from build123d import *

# Parameters (mm, degrees)
BOSS_EXTRUDE1_DEPTH = 12.5
SKETCH4_OUTSIDE_W   = 62.868
SKETCH4_OUTSIDE_H   = 25.468
SKETCH4_OUTSIDE_R   = 5
CUT_EXTRUDE6_DEPTH  = 9.11
SKETCH5_R           = 3
CUT_EXTRUDE7_DEPTH  = 9.11
CUT_EXTRUDE8_REACH  = 21.017
SKETCH6_R           = 2.5


with BuildPart() as part:
    # Sketch1 → Boss-Extrude1 (new body)
    with BuildSketch(Plane.XY):
        with BuildLine():
            Line((-10.816653826, 19.01731952), (-19.949874371, 19.01731952))
            Line((-19.949874371, 19.01731952), (-24.949874371, 19.01731952))
            Line((-24.949874371, 19.01731952), (-24.949874371, 17.01731952))
            Line((-24.949874371, 17.01731952), (-19.949874371, 17.01731952))
            Line((-19.949874371, 17.01731952), (-12.369316877, 17.01731952))
            ThreePointArc((-12.369316877, 17.01731952), (-11.780968471, 16.82592706), (-11.417830963, 16.325011828))
            ThreePointArc((-11.417830963, 16.325011828), (-8.966906745, 12.042698311), (-5, 9.108607405))
            Line((-5, 9.108607405), (-5, 0))
            Line((-5, 0), (5, 0))
            Line((5, 0), (5, 9.108607405))
            ThreePointArc((5, 9.108607405), (8.966906745, 12.042698311), (11.417830963, 16.325011828))
            ThreePointArc((11.417830963, 16.325011828), (11.780968471, 16.82592706), (12.369316877, 17.01731952))
            Line((12.369316877, 17.01731952), (19.949874371, 17.01731952))
            Line((19.949874371, 17.01731952), (24.949874371, 17.01731952))
            Line((24.949874371, 17.01731952), (24.949874371, 19.01731952))
            Line((24.949874371, 19.01731952), (19.949874371, 19.01731952))
            Line((19.949874371, 19.01731952), (10.816653826, 19.01731952))
            ThreePointArc((10.816653826, 19.01731952), (10.177051677, 18.786025635), (9.83332166, 18.199137702))
            ThreePointArc((9.83332166, 18.199137702), (0, 10.01731952), (-9.83332166, 18.199137702))
            ThreePointArc((-9.83332166, 18.199137702), (-10.177051677, 18.786025635), (-10.816653826, 19.01731952))
        make_face()
    extrude(amount=BOSS_EXTRUDE1_DEPTH)

    # Sketch4 outside → Cut-Extrude6 (cut)
    with BuildSketch(Plane.XZ):
        with Locations((0, 6.25)):
            Rectangle(SKETCH4_OUTSIDE_W, SKETCH4_OUTSIDE_H)
        with Locations((0, 6.25)):
            Circle(SKETCH4_OUTSIDE_R, mode=Mode.SUBTRACT)
    extrude(amount=-CUT_EXTRUDE6_DEPTH, mode=Mode.SUBTRACT)

    # Sketch5 → Cut-Extrude7 (cut)
    with BuildSketch(Plane.XZ):
        with Locations((0, 6.25)):
            Circle(SKETCH5_R)
    extrude(amount=-CUT_EXTRUDE7_DEPTH, mode=Mode.SUBTRACT)

    # Sketch6 → Cut-Extrude8 (cut, up to next)
    with BuildSketch(Plane(origin=(0, 19.01731952, 0), x_dir=(1, 0, 0), z_dir=(0, 1, 0)), mode=Mode.PRIVATE) as cut_extrude8_sk1:
        with Locations((-18.699874371, -6.25)):
            Circle(SKETCH6_R)
    cut_extrude8_tool1 = extrude(cut_extrude8_sk1.sketch, amount=-CUT_EXTRUDE8_REACH, mode=Mode.PRIVATE) & part.part
    add(cut_extrude8_tool1.solids().sort_by_distance((-18.699874, 19.01732, 6.25))[0], mode=Mode.SUBTRACT)
    # Sketch6 → Cut-Extrude8 (cut, up to next)
    with BuildSketch(Plane(origin=(0, 19.01731952, 0), x_dir=(1, 0, 0), z_dir=(0, 1, 0)), mode=Mode.PRIVATE) as cut_extrude8_sk2:
        with Locations((18.699874371, -6.25)):
            Circle(SKETCH6_R)
    cut_extrude8_tool2 = extrude(cut_extrude8_sk2.sketch, amount=-CUT_EXTRUDE8_REACH, mode=Mode.PRIVATE) & part.part
    add(cut_extrude8_tool2.solids().sort_by_distance((18.699874, 19.01732, 6.25))[0], mode=Mode.SUBTRACT)


solid = part.part
The model under review builds one solid part; all positions refer to its coordinate system, in mm. A direction names the side the tool comes from. Give positions to 0.01 mm unless a question says otherwise; leave off trailing zeros. Write each loop counter-clockwise with the first axis right and the second up, starting at its lowest first coordinate (ties: lowest second). Pieces come first, ordered by that corner, then holes.
1. Add section A-A, the plane z = 6.25. Count the separate pieces of the cut face and the enclosed holes in it, plus the area to 3 significant figures.
2. For P1, Ø4, axis at x = -19, z = 8, coming from the -Y side; P2, Ø5, axis at x = 0, z = 6.25, coming from the -Y side, all flat-tipped, find the tip position at first contact; note any pin that passes through.
3. Add section D-D, the plane y = 8.25. Write out the cut boundary in (x, z).
4. Draft analysis for pull direction X (two halves, no side actions). For faces 4 (the flat face through (19, 17.017, 3)), 5 (the cylindrical face through (21.01, 18.03, 7.21)), 6 (the cylindrical face through (-0.65, 4.49, 3.32)), 7 (the flat face through (-24.95, 18, 6)), state which applies: +X half, -X half, draft (parallel to the pull), parting line (faces both ways), or undercut.
5. Add section B-B, the plane x = 0. Write out the cut boundary in (y, z).
6. Add section C-C, the plane x = 18. Write out the cut boundary in (y, z).
7. Tool access review of faces 1 (the flat face through (-19, 17.017, 3)), 2 (the cylindrical face through (-1.08, 4.49, 1.37)), 3 (the cylindrical face through (-10.17, 18.78, 6.16)): name each direction out of +Z, -Z, +X, -X, +Y, -Y from which nothing blocks a thin tool from reaching the whole face with its end or side.
8. Wall thickness on L1, parallel to Z at x = 0, y = 4.75; L2, parallel to Y at x = 20, z = 2.75; L3, parallel to X at y = 17.45, z = 6.25: over which ranges is each line inside the solid? List them lowest first.
Worked answers:
1. separate pieces: 3
1. enclosed holes: 0
1. area: 127 mm2
2. P1: stops at y = 17.02
2. P2: stops at y = 9.11
3. outline: circle Ø10 at (0, 6.25); hole circle Ø6 at (0, 6.25)
4. face 4: draft
4. face 5: undercut
4. face 6: undercut
4. face 7: -X half
5. outline: (0, 1.25) - (9.11, 1.25) - (9.11, 0) - (10.02, 0) - (10.02, 12.5) - (9.11, 12.5) - (9.11, 11.25) - (0, 11.25) - (0, 9.25) - (9.11, 9.25) - (9.11, 3.25) - (0, 3.25) - close
6. outline: (17.02, 0) - (19.02, 0) - (19.02, 3.85) - (17.02, 3.85) - close; (17.02, 8.65) - (19.02, 8.65) - (19.02, 12.5) - (17.02, 12.5) - close
7. face 1: +Z, -Z, -X, -Y
7. face 2: -Y
7. face 3: +Z, -Z, +Y
8. L1: z = 1.25 to 3.25, 9.25 to 11.25
8. L2: y = 17.02 to 19.02
8. L3: x = -24.95 to -21.2, -16.2 to -9.66, 9.66 to 16.2, 21.2 to 24.95
